from build123d import *

# Parameters (mm, degrees)
F2_R     = 7
F3_R     = 23.533943
F4_DEPTH = 23.2
F5_R     = 4


with BuildPart() as f1:
    # F0 (on Front) → F1 (revolve)
    with BuildSketch(Plane.XZ):
        with BuildLine():
            Line((-30.5, -54.3), (0, -54.3))
            Line((0, -54.3), (0, 54.3))
            Line((0, 54.3), (-23.5, 54.3))
            ThreePointArc((-23.5, 54.3), (-28.449747, 52.249747), (-30.5, 47.3))
            Line((-30.5, 47.3), (-30.5, -54.3))
        make_face()
    revolve(axis=Axis((0, 0, 0), (0, 0, -1)))

    # F2
    f2_edges = [f1.edges().sort_by_distance(p)[0] for p in [
        (30.5, 0, -54.3),
    ]]
    fillet(f2_edges, radius=F2_R)

    # F3 (on face) → F4 (join)
    with BuildSketch(Plane.XY.offset(54.3)):
        Circle(F3_R)
    extrude(amount=F4_DEPTH)

    # F5
    f5_edges = [f1.edges().sort_by_distance(p)[0] for p in [
        (-23.533943, 0, 77.5),
    ]]
    fillet(f5_edges, radius=F5_R)


solid = f1.part
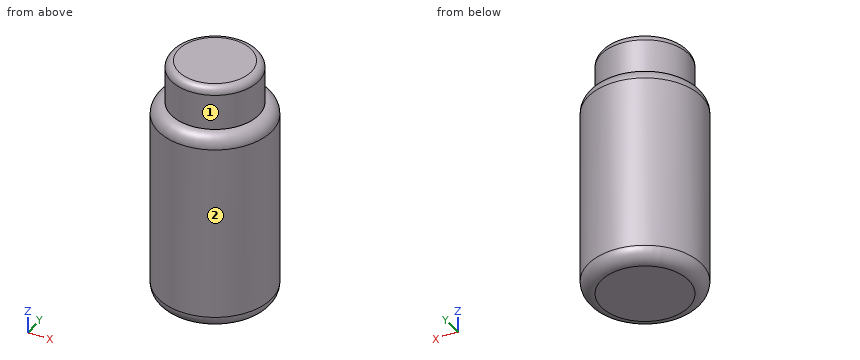
Could you check a few things on this model? Use its own coordinates, in mm. Face numbers are marked on the shaded views. A direction names the side the tool comes from. Coordinates: 2 decimals unless noted, no trailing zeros. Loops run counter-clockwise (first coordinate to the right, second up) from the corner with the lowest first, then second, coordinate; pieces in that order, holes last. Notation, with made-up numbers: (33.25, 22.5) -> (44.25, 22.5) arc R20 ccw to (44.25, 56.5) -> close; hole circle Ø2 at (36.25, -29). An arc over 180 degrees is marked (long way). Answer in a Markdown table with one row per item.
(1) Will these pins go through, and if not, where does the flat tip stop? pin 1 Ø3 at (x, z) = (-15, 46) entering from +Y; pin 2 Ø4 at (y, z) = (9.5, -38.5) entering from -X; pin 3 Ø12 at (y, z) = (3.5, 26) entering from +X; pin 4 Ø8 at (x, z) = (-1.5, 47) entering from -Y.
Results found:
| item | result |
|---|---|
| pin 1 | stops at y = 27.35 |
| pin 2 | stops at x = -29.56 |
| pin 3 | stops at x = 30.5 |
| pin 4 | stops at y = -30.5 |
(2) If I drill on probe 1 along Y at (x, z) = (0, 42); probe 2 along X at (y, z) = (-1, 58); probe 3 along Y at (x, z) = (3, -48), over which ranges is the centre line in solid material (lowest first)?
Results found:
| item | result |
|---|---|
| probe 1 | y = -30.5 to 30.5 |
| probe 2 | x = -23.51 to 23.51 |
| probe 3 | y = -30.32 to 30.32 |
(3) Imagine slicing it at C-C (z = -2.5). List the corners of the cut face in (x, y) for me.
Results found:
| item | result |
|---|---|
| outline | circle Ø61 at (0, 0) |
(4) For the marked faces 1 and 2, which set-ups out of +Z, -Z, +X, -X, +Y, -Y let a thin tool reach every point of the face, with its end or its side?
Results found:
| item | result |
|---|---|
| face 1 | +Z |
| face 2 | +Z, -Z |
